Verification items for the finished model (mm, model axes). Round coordinates to 2 decimals unless told otherwise and drop trailing zeros. Write each loop counter-clockwise with the first axis right and the second up, starting at its lowest first coordinate (ties: lowest second). Pieces come first, ordered by that corner, then holes. Notation, with made-up numbers: (-29, -8.75) - (2, -8.75) arc R21 ccw to (2, 4.25) - close; hole circle Ø4 at (55, 17). An arc over 180 degrees is marked (long way). Answer as a JSON object with one key per item and string values.
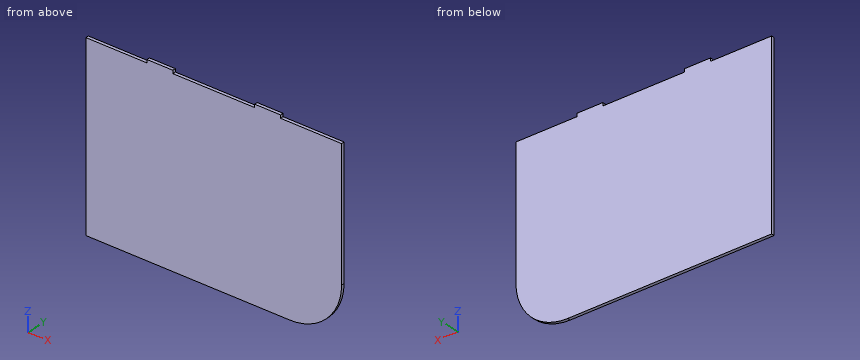
```python
from build123d import *

# Parameters (mm, degrees)
BOSS_EXTRUDE1_DEPTH = 6


with BuildPart() as part:
    # Sketch1 → Boss-Extrude1 (new body)
    with BuildSketch(Plane(origin=(0, 0, 0), x_dir=(1, 0, 0), z_dir=(0, 1, 0))):
        with BuildLine():
            Line((54.064062015, -230.864850181), (54.064062015, -236.864850181))
            Line((54.064062015, -236.864850181), (104.064062015, -236.864850181))
            Line((104.064062015, -236.864850181), (104.064062015, -230.864850181))
            Line((104.064062015, -230.864850181), (222.064062015, -230.864850181))
            Line((222.064062015, -230.864850181), (222.064062015, 19.135149819))
            ThreePointArc((222.064062015, 19.135149819), (192.774740133, 89.845827938), (122.064062015, 119.135149819))
            Line((122.064062015, 119.135149819), (-271.935937985, 119.135149819))
            Line((-271.935937985, 119.135149819), (-271.935937985, -230.864850181))
            Line((-271.935937985, -230.864850181), (-153.935937985, -230.864850181))
            Line((-153.935937985, -230.864850181), (-153.935937985, -236.864850181))
            Line((-153.935937985, -236.864850181), (-103.935937985, -236.864850181))
            Line((-103.935937985, -236.864850181), (-103.935937985, -230.864850181))
            Line((-103.935937985, -230.864850181), (54.064062015, -230.864850181))
        make_face()
    extrude(amount=BOSS_EXTRUDE1_DEPTH)


solid = part.part
```
1. Cross-section at A-A (y = 3.6). Record the boundary of the cut face in (x, z).
Completed:
{"outline": "(-271.94, -119.14) - (122.06, -119.14) arc R100 ccw to (222.06, -19.14) - (222.06, 230.86) - (104.06, 230.86) - (104.06, 236.86) - (54.06, 236.86) - (54.06, 230.86) - (-103.94, 230.86) - (-103.94, 236.86) - (-153.94, 236.86) - (-153.94, 230.86) - (-271.94, 230.86) - close"}
2. Material ranges on probe 1 along Z at (x, y) = (-175.5, 1.4); probe 2 along X at (y, z) = (1.1, -104.5); probe 3 along X at (y, z) = (4.55, -38), recorded low to high. Write a range as from..to.
Completed:
{"probe 1": "z = -119.14..230.86", "probe 2": "x = -271.94..174.15", "probe 3": "x = -271.94..220.27"}
3. Go/stop test with flat-tipped pins: pin 1 (3 mm diameter, centred on y = 2.5, z = 235, fed in from -X); pin 2 (1 mm diameter, centred on x = -178.5, y = 0.5, fed in from +Z); pin 3 (3 mm diameter, centred on y = 4, z = 234, fed in from +X); pin 4 (3 mm diameter, centred on x = -45, z = 190.5, fed in from -Y). Record where each tip stops, or that it passes through.
Completed:
{"pin 1": "stops at x = -153.94", "pin 2": "stops at z = 230.86", "pin 3": "stops at x = 104.06", "pin 4": "stops at y = 0"}
4. Cross-section at B-B (x = 11). Record the boundary of the cut face in (y, z).
Completed:
{"outline": "(0, -119.14) - (6, -119.14) - (6, 230.86) - (0, 230.86) - close"}
